Verification items for this drawing (mm, ordinates from the low corner). Round coordinates to 2 decimals unless told otherwise and drop trailing zeros. Order: outer loops, then holes, each group sorted by start corner. A loop starts at its lowest first (then second) coordinate and runs counter-clockwise, first axis right, second up. Notation, with made-up numbers: (-13, -36.5) - (27, -36.5) arc R24 ccw to (27, -16.5) - close; hole circle Ø2 at (-12, -40). An arc over 180 degrees is marked (long way). Answer as CSV lines item,"result". Start each with the question number.
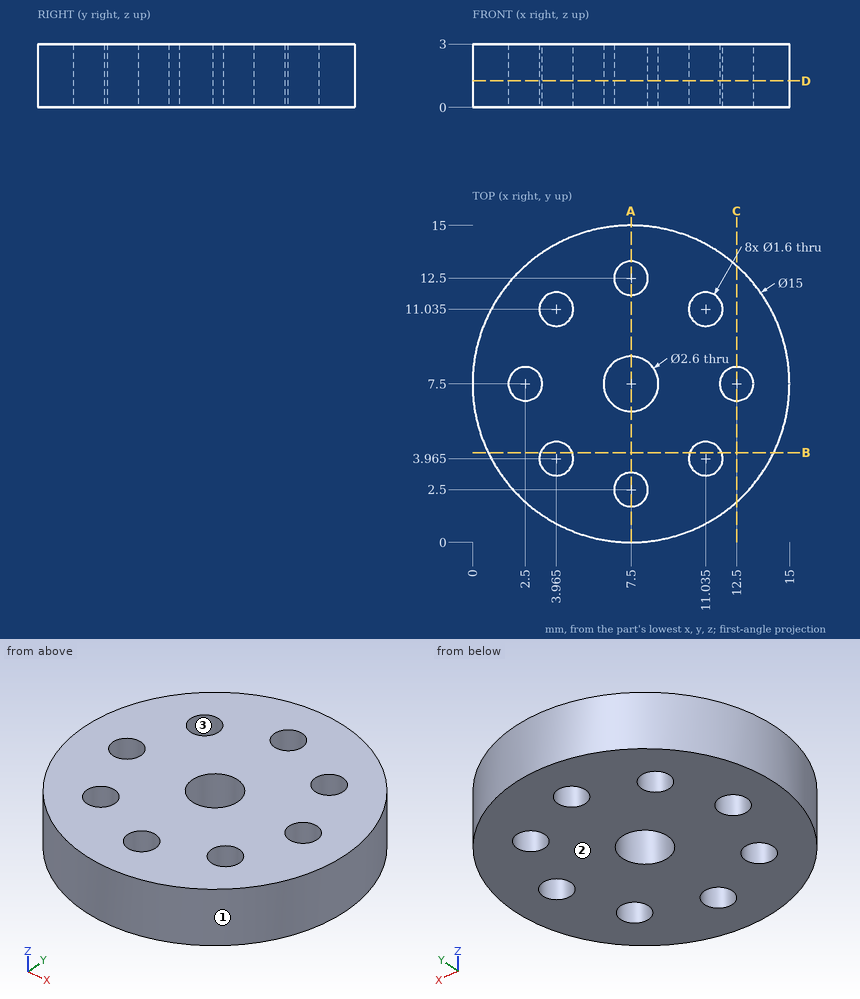
1. Section check B-B on y = 4.25. Record the boundary of the cut face in (x, z).
2. Section check A-A on x = 7.5. Record the boundary of the cut face in (y, z), plus the area to 3 significant figures.
3. Thickness scan on probe 1 along Y at (x, z) = (7.5, 1.2); probe 2 along Y at (x, z) = (2, 1.95) (1 decimal); probe 3 along Y at (x, z) = (2.75, 1.7) (1 decimal). Record the ranges inside material, lowest first.
4. Section check D-D on z = 1.25. Count the separate pieces of the cut face and the enclosed holes in it, plus the area to 3 significant figures.
5. Section check C-C on x = 12.5. Record the boundary of the cut face in (y, z).
6. Draft check along X on the marked faces 1, 2 and 3. Enter one of: released by +X, released by -X, zero draft, split by the parting line, or undercut.
7. Go/stop test with flat-tipped pins: pin 1 Ø1.8 at (x, y) = (11.04, 11.04) entering from +Z; pin 2 Ø1 at (x, z) = (11.5, 2.5) entering from -Y. Record where each tip stops, or that it passes through.
Numbers:
1,outline,"(0.74, 0) - (3.22, 0) - (3.22, 3) - (0.74, 3) - close; (4.71, 0) - (10.29, 0) - (10.29, 3) - (4.71, 3) - close; (11.78, 0) - (14.26, 0) - (14.26, 3) - (11.78, 3) - close"
2,outline,"(0, 0) - (1.7, 0) - (1.7, 3) - (0, 3) - close; (3.3, 0) - (6.2, 0) - (6.2, 3) - (3.3, 3) - close; (8.8, 0) - (11.7, 0) - (11.7, 3) - (8.8, 3) - close; (13.3, 0) - (15, 0) - (15, 3) - (13.3, 3) - close"
2,area,"27.6 mm2"
3,probe 1,"y = 0 to 1.7, 3.3 to 6.2, 8.8 to 11.7, 13.3 to 15"
3,probe 2,"y = 2.4 to 6.9, 8.1 to 12.6"
3,probe 3,"y = 1.7 to 6.7, 8.3 to 13.3"
4,separate pieces,"1"
4,enclosed holes,"9"
4,area,"155 mm2"
5,outline,"(1.91, 0) - (6.7, 0) - (6.7, 3) - (1.91, 3) - close; (8.3, 0) - (13.09, 0) - (13.09, 3) - (8.3, 3) - close"
6,face 1,"split by the parting line"
6,face 2,"zero draft"
6,face 3,"undercut"
7,pin 1,"stops at z = 3"
7,pin 2,"stops at y = 0.87"
